Geometry: final body of the model. Coordinates: model frame, mm. A direction names the side the tool comes from. Coordinates: 2 decimals unless noted, no trailing zeros. Order: outer loops, then holes, each group sorted by start corner. A loop starts at its lowest first (then second) coordinate and runs counter-clockwise, first axis right, second up. Notation, with made-up numbers: (8.25, 64) -> (15.25, 64) arc R22 ccw to (15.25, 86) -> close; hole circle Ø8 at (73.5, -22). An arc over 180 degrees is marked (long way). Use one line per item in the form item = value.
```python
from build123d import *

# Parameters (mm, degrees)
F1_DEPTH = 40
F3_DEPTH = 22.5
F5_DEPTH = 15
F6_R     = 3
F7_DEPTH = 1
F8_W     = 23.385154
F8_H     = 40.474307
F9_DEPTH = 1


with BuildPart() as f1:
    # F0 (on Right) → F1 (new body, symmetric)
    with BuildSketch(Plane.YZ):
        Polygon((35.49702, 43.180404), (-34.50298, 43.180404), (-45.997234, -6.819596), (-85.997234, -6.819596), (-85.997234, -36.819596), (35.49702, -36.819596), align=None)
    extrude(amount=F1_DEPTH, both=True)

    # F2 (on Right) → F3 (join, symmetric)
    with BuildSketch(Plane.YZ):
        Polygon((35.575308, 43.072656), (35.575308, 33.278871), (43.969978, 51.067576), (32.577209, 51.067576), (23.383051, 43.072656), align=None)
    extrude(amount=F3_DEPTH, both=True)

    # F4 (on Right) → F5 (join, symmetric)
    with BuildSketch(Plane.YZ):
        Polygon((-74.98049, -6.83292), (-50.600782, -6.762254), (-69.539219, 0), align=None)
    extrude(amount=F5_DEPTH, both=True)

    # F6 (on face) → F7 (cut)
    with BuildSketch(Plane(origin=(0, -42.553907, 33.887025), x_dir=(1, 0, 0), z_dir=(0, -0.782267, 0.622944))):
        with Locations((-8, -47.068199)):
            Circle(F6_R)
        with Locations((8.026602, -47.068199)):
            Circle(F6_R)
    extrude(amount=-F7_DEPTH, mode=Mode.SUBTRACT)

    # F8 (on face) → F9 (cut)
    with BuildSketch(Plane.YZ.offset(40)):
        Polygon((-4.19944, 40.474307), (-30.382816, 40.474307), (-39.687255, 0), (-13.393601, 0), align=None)
        with Locations((17.28692, 20.237153)):
            Rectangle(F8_W, F8_H)
    extrude(amount=-F9_DEPTH, mode=Mode.SUBTRACT)


solid = f1.part
```
1) Section C-C, the plane z = -12. Output: boundary loops of the cut face in (x, y), and give its area (3 significant figures).
Results found:
outline = (-40, -86) -> (40, -86) -> (40, 35.5) -> (-40, 35.5) -> close
area = 9,720 mm2
2) Section A-A, the plane x = 1.5. Output: boundary loops of the cut face in (y, z), and give its area (3 significant figures).
Results found:
outline = (-86, -36.82) -> (35.5, -36.82) -> (35.5, 43.07) -> (35.58, 43.07) -> (35.58, 33.28) -> (43.97, 51.07) -> (32.58, 51.07) -> (23.51, 43.18) -> (-34.5, 43.18) -> (-46, -6.82) -> (-70.38, -6.82) -> (-50.6, -6.76) -> (-69.54, 0) -> (-74.97, -6.82) -> (-86, -6.82) -> close
area = 7,650 mm2
3) Material intervals for probe 1 along Z at (x, y) = (-29, -49); probe 2 along Z at (x, y) = (28, -31.5); probe 3 along X at (y, z) = (27, 25.5), sorted ascending. Write a range as from..to.
Results found:
probe_1 = -36.82..-6.82
probe_2 = -36.82..43.18
probe_3 = -40..39
4) Access query for faces 1 (the flat face through (0.21, -59.937, -3.428)), 2 (the flat face through (-15, -66, -5)), 3 (the flat face through (39, -22, 21)), 4 (the flat face through (7.985, -71.066, -3.523)). Directions: +Z, -Z, +X, -X, +Y, -Y. A direction counts if a zero-diameter tool reaches every point of the face in a straight line with its end or side. Return the directions, or none.
Results found:
face_1 = +Z, +X, -X
face_2 = +Z, -X, -Y
face_3 = +X
face_4 = none
5) Contact query for flat-ended pins moving along their axis: P1, Ø0.8, axis at x = 39.5, z = 22.5, coming from the -Y side; P2, Ø0.8, axis at x = 39.5, y = -32, coming from the +Z side; P3, Ø1.1, axis at x = 39.5, z = 27.5, coming from the +Y side. Output: stop coordinate, or through.
Results found:
P1 = -39.35
P2 = 43.18
P3 = 35.5
6) Section D-D, the plane y = 25.5. Output: boundary loops of the cut face in (x, z).
Results found:
outline = (-40, -36.82) -> (40, -36.82) -> (40, 0) -> (39, 0) -> (39, 40.47) -> (40, 40.47) -> (40, 43.18) -> (22.5, 43.18) -> (22.5, 44.91) -> (-22.5, 44.91) -> (-22.5, 43.18) -> (-40, 43.18) -> close
7) Section B-B, the plane y = -58.5. Output: boundary loops of the cut face in (x, z).
Results found:
outline = (-40, -36.82) -> (40, -36.82) -> (40, -6.82) -> (-40, -6.82) -> close; (-15, -6.79) -> (15, -6.79) -> (15, -3.94) -> (-15, -3.94) -> close
8) Pull-direction query (Y, two-part tool) for faces 5 (the flat face through (0.315, 39.714, 42.049)), 6 (the flat face through (39, 17, 21)), 7 (the flat face through (-40, -13, -5)); classes: released by +Y, released by -Y, zero draft, split by the parting line, or undercut.
Results found:
face_5 = released by +Y
face_6 = undercut
face_7 = zero draft
